Input: dimensioned drawing with shaded views. Units: mm. Origin: part minimum x, y, z. Coordinates: 2 decimals unless noted, no trailing zeros. Order: outer loops, then holes, each group sorted by start corner. A loop starts at its lowest first (then second) coordinate and runs counter-clockwise, first axis right, second up. Notation, with made-up numbers: (66.5, -21) -> (93.5, -21) arc R22 ccw to (93.5, 1) -> close; hole circle Ø4 at (36, 34.25). An arc over 180 degrees is marked (long way). Answer in a Markdown table with one row per item. Add a question column.
1) Section query D-D on y = 4. Return the cut outline in (x, z).
2) Section query C-C on y = 9.25. Return the cut outline in (x, z), then the cut area to 3 significant figures.
3) Pull-direction query (Y, two-part tool) for the marked faces 1, 2 and 3; classes: +Y half, -Y half, draft (parallel to the pull), parting line (faces both ways), or undercut.
4) Section query B-B on x = 7.5. Return the cut outline in (y, z).
5) Contact query for flat-ended pins moving along their axis: P1, Ø6, axis at x = 3.5, y = 9, coming from the +Z side; P2, Ø4, axis at x = 10, y = 2, coming from the +Z side; P3, Ø4, axis at x = 3.5, y = 10, coming from the +Z side. Output: stop coordinate, or through.
6) Section query A-A on z = 7.5. Return the cut outline in (x, y).
7) Ray query, line 1 (Z direction, x = 4.5, y = 8.75); line 2 (X direction, y = 6.25, z = 8.25); line 3 (Z direction, x = 2, y = 8.5). Return the intervals inside material, ascending. Write a range as from..to.
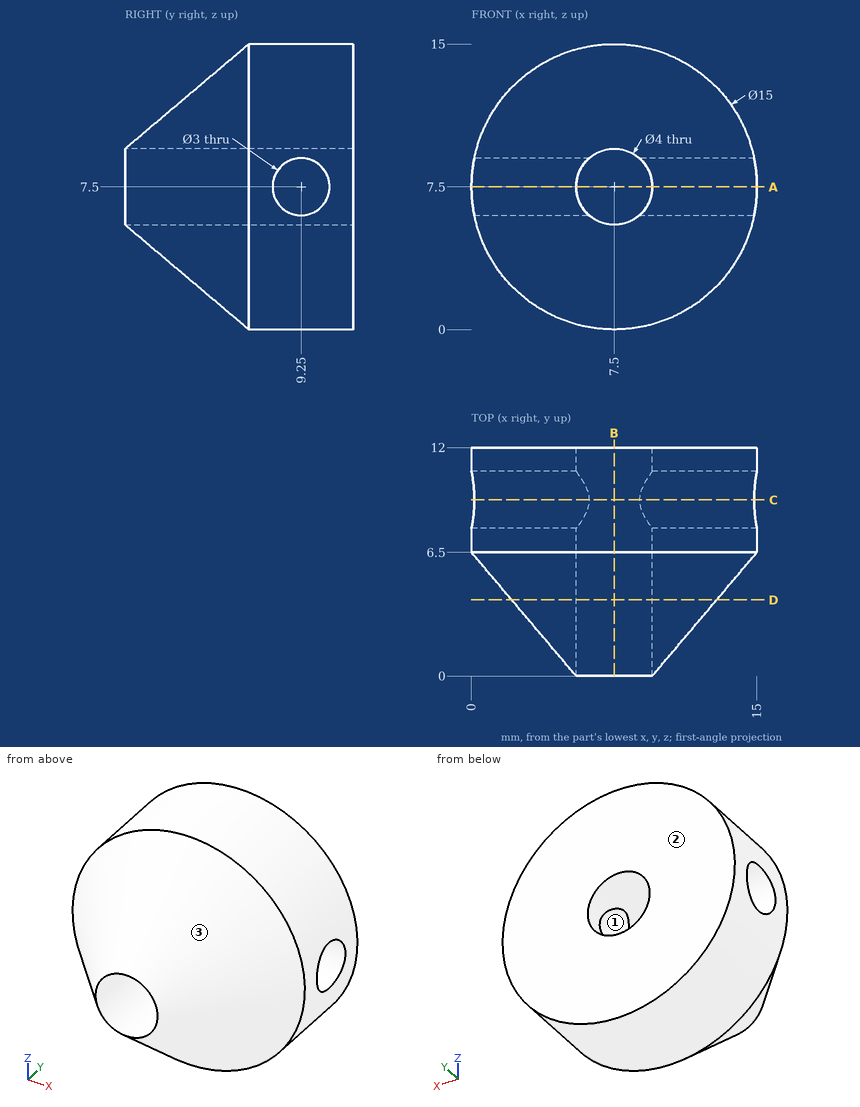
Result:
| question | item | result |
|---|---|---|
| 1 | outline | circle Ø10.77 at (7.5, 7.5); hole circle Ø4 at (7.5, 7.5) |
| 2 | outline | (0.15, 6) arc R7.5 ccw to (14.85, 6) -> (8.82, 6) arc R2 cw to (6.18, 6) -> close; (0.15, 9) -> (6.18, 9) arc R2 cw to (8.82, 9) -> (14.85, 9) arc R7.5 ccw to start |
| 2 | area | 130 mm2 |
| 3 | face 1 | undercut |
| 3 | face 2 | +Y half |
| 3 | face 3 | -Y half |
| 4 | outline | (0, 5.5) -> (6.5, 0) -> (12, 0) -> (12, 5.5) -> close; (0, 9.5) -> (12, 9.5) -> (12, 15) -> (6.5, 15) -> close |
| 5 | P1 | z = 14.93 |
| 5 | P2 | z = 12.46 |
| 5 | P3 | z = 14.73 |
| 6 | outline | (0, 6.5) -> (5.5, 0) -> (5.5, 7.75) -> (0, 7.75) -> close; (0, 10.75) -> (5.5, 10.75) -> (5.5, 12) -> (0, 12) -> close; (9.5, 0) -> (15, 6.5) -> (15, 7.75) -> (9.5, 7.75) -> close; (9.5, 10.75) -> (15, 10.75) -> (15, 12) -> (9.5, 12) -> close |
| 7 | line 1 | 0.63..6.09, 8.91..14.37 |
| 7 | line 2 | 0.25..5.65, 9.35..14.75 |
| 7 | line 3 | 2.4..6.2, 8.8..12.6 |
